```python
from build123d import *

# Parameters (mm, degrees)
EXTRUDE_1_DEPTH      = 148
SKETCH_2_W           = 144
SKETCH_2_H           = 74
CUT_EXTRUDE_1_DEPTH  = 8
SKETCH_3_W           = 144
SKETCH_3_H           = 76
CUT_EXTRUDE_2_DEPTH  = 17.5
SKETCH_6_R           = 1.525
EXTRUDE_2_DEPTH      = 2
SKETCH_7_R           = 1.525
CUT_EXTRUDE_3_DEPTH  = 2
SKETCH_8_W           = 100
SKETCH_8_H           = 10
CUT_EXTRUDE_4_DEPTH  = 1
SKETCH_10_R          = 1.5
SKETCH_10_R_2        = 2
CUT_EXTRUDE_6_DEPTH  = 2
SKETCH_12_W          = 43
SKETCH_12_H          = 5
SKETCH_12_W_2        = 25
SKETCH_12_H_2        = 6
CUT_EXTRUDE_7_DEPTH  = 2
SKETCH_14_R          = 1.525
CUT_EXTRUDE_8_DEPTH  = 2
SKETCH_15_W          = 8
SKETCH_15_H          = 8
CUT_EXTRUDE_9_DEPTH  = 10
CUT_EXTRUDE_11_DEPTH = 10
EXTRUDE_START        = 48
EXTRUDE_3_DEPTH      = 15
FILLET_1_R           = 1
FILLET_2_R           = 1


with BuildPart() as part:
    # 草图1 → 凸台-拉伸1 (new body)
    with BuildSketch(Plane(origin=(0, 0, 0), x_dir=(0, 0, -1), z_dir=(1, 0, 0))):
        Polygon((0, 0), (154, 0), (154, 19.5), (76, 19.5), (76, 9.5), (0, 9.5), align=None)
    extrude(amount=EXTRUDE_1_DEPTH)

    # 草图2 → 切除-拉伸1 (cut)
    with BuildSketch(Plane(origin=(0, 9.5, 0), x_dir=(1, 0, 0), z_dir=(0, 1, 0))):
        with Locations((74, 39)):
            Rectangle(SKETCH_2_W, SKETCH_2_H)
    extrude(amount=-CUT_EXTRUDE_1_DEPTH, mode=Mode.SUBTRACT)

    # 草图3 → 切除-拉伸2 (cut)
    with BuildSketch(Plane.XZ):
        with Locations((74, -114)):
            Rectangle(SKETCH_3_W, SKETCH_3_H)
    extrude(amount=-CUT_EXTRUDE_2_DEPTH, mode=Mode.SUBTRACT)

    # 草图6 → 凸台-拉伸2 (add)
    # profile 1 of 4: a face of its own
    with BuildSketch(Plane(origin=(0, 9.5, 0), x_dir=(1, 0, 0), z_dir=(0, 1, 0))):
        with BuildLine():
            Line((146, 5), (156, 5))
            ThreePointArc((156, 5), (161, 10), (156, 15))
            Line((156, 15), (146, 15))
            Line((146, 15), (146, 5))
        make_face()
        with Locations(Location((156, 10, 0), (0, 0, 270))):
            Circle(SKETCH_6_R, mode=Mode.SUBTRACT)
    # profile 2 of 4: a face of its own
    with BuildSketch(Plane(origin=(0, 9.5, 0), x_dir=(1, 0, 0), z_dir=(0, 1, 0))):
        with BuildLine():
            Line((-8, 15), (2, 15))
            Line((2, 15), (2, 5))
            Line((2, 5), (-8, 5))
            ThreePointArc((-8, 5), (-13, 10), (-8, 15))
        make_face()
        with Locations(Location((-8, 10, 0), (0, 0, 90))):
            Circle(SKETCH_6_R, mode=Mode.SUBTRACT)
    # profile 3 of 4: a face of its own
    with BuildSketch(Plane(origin=(0, 9.5, 0), x_dir=(1, 0, 0), z_dir=(0, 1, 0))):
        with BuildLine():
            Line((146, 139), (156, 139))
            ThreePointArc((156, 139), (161, 144), (156, 149))
            Line((156, 149), (146, 149))
            Line((146, 149), (146, 139))
        make_face()
        with Locations(Location((156, 144, 0), (0, 0, 270))):
            Circle(SKETCH_6_R, mode=Mode.SUBTRACT)
    # profile 4 of 4: a face of its own
    with BuildSketch(Plane(origin=(0, 9.5, 0), x_dir=(1, 0, 0), z_dir=(0, 1, 0))):
        with BuildLine():
            Line((-8, 149), (2, 149))
            Line((2, 149), (2, 139))
            Line((2, 139), (-8, 139))
            ThreePointArc((-8, 139), (-13, 144), (-8, 149))
        make_face()
        with Locations(Location((-8, 144, 0), (0, 0, 90))):
            Circle(SKETCH_6_R, mode=Mode.SUBTRACT)
    extrude(amount=EXTRUDE_2_DEPTH)

    # 草图7 → 切除-拉伸3 (cut)
    with BuildSketch(Plane(origin=(0, 19.5, 0), x_dir=(1, 0, 0), z_dir=(0, 1, 0))):
        with Locations(Location((118, 80, 0), (0, 0, 270))):
            Circle(SKETCH_7_R)
        with Locations(Location((30, 80, 0), (0, 0, 270))):
            Circle(SKETCH_7_R)
    extrude(amount=-CUT_EXTRUDE_3_DEPTH, mode=Mode.SUBTRACT)

    # 草图8 → 切除-拉伸4 (cut)
    with BuildSketch(Plane(origin=(0, 19.5, 0), x_dir=(1, 0, 0), z_dir=(0, 1, 0))):
        with Locations((74, 81)):
            Rectangle(SKETCH_8_W, SKETCH_8_H)
    extrude(amount=-CUT_EXTRUDE_4_DEPTH, mode=Mode.SUBTRACT)

    # 草图10 → 切除-拉伸6 (cut)
    with BuildSketch(Plane(origin=(0, 19.5, 0), x_dir=(1, 0, 0), z_dir=(0, 1, 0))):
        with Locations((92.824957671, 0)):
            Circle(SKETCH_10_R)
        with Locations(Location((87.811120796, 135.911745597, 0), (0, 0, 270))):
            Circle(SKETCH_10_R_2)
        with Locations(Location((95.811120796, 135.911745597, 0), (0, 0, 270))):
            Circle(SKETCH_10_R_2)
        with Locations(Location((103.811120796, 135.911745597, 0), (0, 0, 270))):
            Circle(SKETCH_10_R_2)
        with Locations(Location((111.811120796, 135.911745597, 0), (0, 0, 270))):
            Circle(SKETCH_10_R_2)
        with Locations(Location((119.811120796, 135.911745597, 0), (0, 0, 270))):
            Circle(SKETCH_10_R_2)
        with Locations(Location((127.811120796, 135.911745597, 0), (0, 0, 270))):
            Circle(SKETCH_10_R_2)
        with Locations(Location((95.811120796, 127.911745597, 0), (0, 0, 270))):
            Circle(SKETCH_10_R_2)
        with Locations(Location((103.811120796, 127.911745597, 0), (0, 0, 270))):
            Circle(SKETCH_10_R_2)
        with Locations(Location((111.811120796, 127.911745597, 0), (0, 0, 270))):
            Circle(SKETCH_10_R_2)
        with Locations(Location((119.811120796, 127.911745597, 0), (0, 0, 270))):
            Circle(SKETCH_10_R_2)
        with Locations(Location((127.811120796, 127.911745597, 0), (0, 0, 270))):
            Circle(SKETCH_10_R_2)
        with Locations(Location((95.811120796, 119.911745597, 0), (0, 0, 270))):
            Circle(SKETCH_10_R_2)
        with Locations(Location((103.811120796, 119.911745597, 0), (0, 0, 270))):
            Circle(SKETCH_10_R_2)
        with Locations(Location((111.811120796, 119.911745597, 0), (0, 0, 270))):
            Circle(SKETCH_10_R_2)
        with Locations(Location((119.811120796, 119.911745597, 0), (0, 0, 270))):
            Circle(SKETCH_10_R_2)
        with Locations(Location((127.811120796, 119.911745597, 0), (0, 0, 270))):
            Circle(SKETCH_10_R_2)
        with Locations(Location((95.811120796, 111.911745597, 0), (0, 0, 270))):
            Circle(SKETCH_10_R_2)
        with Locations(Location((103.811120796, 111.911745597, 0), (0, 0, 270))):
            Circle(SKETCH_10_R_2)
        with Locations(Location((111.811120796, 111.911745597, 0), (0, 0, 270))):
            Circle(SKETCH_10_R_2)
        with Locations(Location((119.811120796, 111.911745597, 0), (0, 0, 270))):
            Circle(SKETCH_10_R_2)
        with Locations(Location((127.811120796, 111.911745597, 0), (0, 0, 270))):
            Circle(SKETCH_10_R_2)
        with Locations(Location((95.811120796, 103.911745597, 0), (0, 0, 270))):
            Circle(SKETCH_10_R_2)
        with Locations(Location((103.811120796, 103.911745597, 0), (0, 0, 270))):
            Circle(SKETCH_10_R_2)
        with Locations(Location((111.811120796, 103.911745597, 0), (0, 0, 270))):
            Circle(SKETCH_10_R_2)
        with Locations(Location((119.811120796, 103.911745597, 0), (0, 0, 270))):
            Circle(SKETCH_10_R_2)
        with Locations(Location((127.811120796, 103.911745597, 0), (0, 0, 270))):
            Circle(SKETCH_10_R_2)
        with Locations(Location((87.811120796, 127.911745597, 0), (0, 0, 270))):
            Circle(SKETCH_10_R_2)
        with Locations(Location((87.811120796, 119.911745597, 0), (0, 0, 270))):
            Circle(SKETCH_10_R_2)
        with Locations(Location((87.811120796, 111.911745597, 0), (0, 0, 270))):
            Circle(SKETCH_10_R_2)
        with Locations(Location((87.811120796, 103.911745597, 0), (0, 0, 270))):
            Circle(SKETCH_10_R_2)
        with BuildLine():
            Line((36.136845643, 134.865517695), (22.562000425, 120.17798634))
            ThreePointArc((22.562000425, 120.17798634), (19.735762768, 120.066717726), (19.624494154, 122.892955383))
            Line((19.624494154, 122.892955383), (33.199339372, 137.580486739))
            ThreePointArc((33.199339372, 137.580486739), (36.025577029, 137.691755353), (36.136845643, 134.865517695))
        make_face()
        with BuildLine():
            Line((52.189559598, 134.554261075), (25.039869163, 105.179198365))
            ThreePointArc((25.039869163, 105.179198365), (22.213631506, 105.067929751), (22.102362892, 107.894167408))
            Line((22.102362892, 107.894167408), (49.252053327, 137.269230119))
            ThreePointArc((49.252053327, 137.269230119), (52.078290985, 137.380498733), (52.189559598, 134.554261075))
        make_face()
        with BuildLine():
            Line((50.824376998, 121.290672478), (37.249531781, 106.603141122))
            ThreePointArc((37.249531781, 106.603141122), (37.360800394, 103.776903465), (40.187038052, 103.888172079))
            Line((40.187038052, 103.888172079), (53.761883269, 118.575703434))
            ThreePointArc((53.761883269, 118.575703434), (53.650614655, 121.401941091), (50.824376998, 121.290672478))
        make_face()
    extrude(amount=-CUT_EXTRUDE_6_DEPTH, mode=Mode.SUBTRACT)

    # 草图12 → 切除-拉伸7 (cut)
    with BuildSketch(Plane(origin=(0, 0, -154), x_dir=(-1, 0, 0), z_dir=(0, 0, -1))):
        with Locations((-97, 4.5)):
            Rectangle(SKETCH_12_W, SKETCH_12_H)
        with Locations((-18, 5)):
            Rectangle(SKETCH_12_W_2, SKETCH_12_H_2)
    extrude(amount=-CUT_EXTRUDE_7_DEPTH, mode=Mode.SUBTRACT)

    # 草图14 → 切除-拉伸8 (cut)
    with BuildSketch(Plane.XZ.offset(-17.5)):
        with Locations(Location((141.5, -80, 0), (0, 0, 270))):
            Circle(SKETCH_14_R)
        with Locations(Location((141.5, -136, 0), (0, 0, 270))):
            Circle(SKETCH_14_R)
        with Locations(Location((7, -136, 0), (0, 0, 270))):
            Circle(SKETCH_14_R)
        with Locations(Location((7, -80, 0), (0, 0, 270))):
            Circle(SKETCH_14_R)
    extrude(amount=-CUT_EXTRUDE_8_DEPTH, mode=Mode.SUBTRACT)

    # 草图15 → 切除-拉伸9 (cut)
    with BuildSketch(Plane(origin=(0, 0, -2), x_dir=(-1, 0, 0), z_dir=(0, 0, -1))):
        with Locations((-41.5, 5.5)):
            Rectangle(SKETCH_15_W, SKETCH_15_H)
        with Locations((-63.5, 5.5)):
            Rectangle(SKETCH_15_W, SKETCH_15_H)
    extrude(amount=-CUT_EXTRUDE_9_DEPTH, mode=Mode.SUBTRACT)

    # 草图16 → 切除-拉伸11 (cut)
    with BuildSketch(Plane(origin=(0, 1.5, 0), x_dir=(1, 0, 0), z_dir=(0, 1, 0))):
        with BuildLine():
            Line((45.5, 2), (45.5, 0))
            Line((45.5, 0), (37.5, 0))
            Line((37.5, 0), (37.5, 2))
            ThreePointArc((37.5, 2), (41.5, 6), (45.5, 2))
        make_face()
        with BuildLine():
            Line((67.5, 2), (67.5, 0))
            Line((67.5, 0), (59.5, 0))
            Line((59.5, 0), (59.5, 2))
            ThreePointArc((59.5, 2), (63.5, 6), (67.5, 2))
        make_face()
    extrude(amount=-CUT_EXTRUDE_11_DEPTH, mode=Mode.SUBTRACT)

    # 草图17 → 凸台-拉伸3 (add)
    with BuildSketch(Plane.XY.offset(-139).offset(EXTRUDE_START)):
        Polygon((148, 14.5), (148, 15.5), (154, 15.5), (154, 9.5), (153, 9.5), (153, 14.5), align=None)
        Polygon((0, 15.5), (-6, 15.5), (-6, 9.5), (-5, 9.5), (-5, 14.5), (0, 14.5), align=None)
    extrude(amount=EXTRUDE_3_DEPTH)

    # 圆角1
    fillet_1_edges = [part.edges().sort_by_distance(p)[0] for p in [
        (-6, 15.5, -83.5),
        (154, 15.5, -83.5),
    ]]
    fillet(fillet_1_edges, radius=FILLET_1_R)

    # 圆角2
    fillet_2_edges = [part.edges().sort_by_distance(p)[0] for p in [
        (-5.5, 9.5, -91),
        (-5.5, 9.5, -76),
        (153.5, 9.5, -91),
        (153.5, 9.5, -76),
    ]]
    fillet(fillet_2_edges, radius=FILLET_2_R)


solid = part.part
```
For this review, take the finished solid that the model builds, in its own axes (mm). A direction names the side the tool comes from. Round coordinates to 2 decimals unless told otherwise and drop trailing zeros. Write each loop counter-clockwise with the first axis right and the second up, starting at its lowest first coordinate (ties: lowest second). Pieces come first, ordered by that corner, then holes. Notation, with made-up numbers: (-33, 10) -> (19, 10) arc R33 ccw to (19, 42) -> close; hole circle Ø5 at (-4, -25). An arc over 180 degrees is marked (long way). One line per question, with ' | ' between items. Start each with the question number.
(1) Mouldability with a two-part tool opening along X and no side actions: class faces 1 (the face through (161, 10, -144)), 2 (the face through (154, 11.5, -144)), 3 (the face through (44.13, 18.51, -114.05)) as released by +X, released by -X, zero draft, split by the parting line, or undercut.
(2) Tool access review of faces 4 (the face through (154, 12, -84)), 5 (the face through (150, 15.5, -84)), 6 (the face through (52, 6, -2)), 7 (the face through (46.88, 18.51, -111.13)): name each direction out of +Z, -Z, +X, -X, +Y, -Y from which nothing blocks a thin tool from reaching the whole face with its end or side.
(3) Add section A-A, the plane x = 63.5. Write out the cut boundary in (y, z), plus the area to 3 significant figures.
(4) Insertion check: P1, Ø4, axis at x = 141.5, z = -136, coming from the -Y side; P2, Ø8, axis at x = 104, y = 14.5, coming from the +Z side; P3, Ø4, axis at x = 151.5, y = 12.5, coming from the -Z side. Each pin has a flat end and moves straight along its axis. Give the tip position at first contact, or say it passes through.
(5) For line 1 along X through (y, z) = (10.95, -10) (3 decimals); line 2 along X through (y, z) = (10.5, -79); line 3 along Z through (x, y) = (111.5, 18.75), list the stretches that pass through material, from the lowest coordinate up. Write a range as from..to.
(6) Add section B-B, the plane z = -40. Write out the cut boundary in (x, y), plus the area to 3 significant figures.
Answer list:
1) face 1: released by +X | face 2: zero draft | face 3: undercut
2) face 4: +X, +Y, -Y | face 5: +Z, -Z, +X, +Y | face 6: +Y | face 7: +Y, -Y
3) outline: (0, -154) -> (19.5, -154) -> (19.5, -86) -> (18.5, -86) -> (18.5, -76) -> (17.5, -76) -> (17.5, -152) -> (0, -152) -> close; (0, -76) -> (1.5, -76) -> (1.5, -6) -> (0, -6) -> close | area: 286 mm²
4) P1: y = 17.5 | P2: z = -76 | P3: z = -149
5) line 1: -13..-9.525, -6.475..2, 146..154.475, 157.525..161 | line 2: -6..-5, 0..2, 146..148, 153..154 | line 3: -154..-137.89, -133.94..-129.89, -125.94..-121.89, -117.94..-113.89, -109.94..-105.89, -101.94..-86
6) outline: (0, 0) -> (148, 0) -> (148, 9.5) -> (146, 9.5) -> (146, 1.5) -> (2, 1.5) -> (2, 9.5) -> (0, 9.5) -> close | area: 254 mm²
